Check sheet for the modelled part. Datum: model origin and axes. Units: mm. A direction names the side the tool comes from. Round coordinates to 2 decimals unless told otherwise and drop trailing zeros. Write each loop counter-clockwise with the first axis right and the second up, starting at its lowest first coordinate (ties: lowest second). Pieces come first, ordered by that corner, then holes. Notation, with made-up numbers: (-22.75, 29.5) -> (34.25, 29.5) arc R10 cw to (34.25, 33.5) -> close; hole circle Ø6 at (82, -40). An arc over 180 degrees is marked (long way). One line per item, written item: value.
from build123d import *

# Parameters (mm, degrees)
SKETCH1_W           = 30
SKETCH1_H           = 100
BOSS_EXTRUDE1_DEPTH = 3.75
CUT_EXTRUDE1_DEPTH  = 6.5


with BuildPart() as part:
    # Sketch1 → Boss-Extrude1 (new, symmetric)
    with BuildSketch(Plane(origin=(0, 0, 0), x_dir=(1, 0, 0), z_dir=(0, 1, 0))):
        with Locations((15, 0)):
            Rectangle(SKETCH1_W, SKETCH1_H)
    extrude(amount=BOSS_EXTRUDE1_DEPTH, both=True)

    # Sketch2 → Cut-Extrude1 (cut)
    with BuildSketch(Plane(origin=(0, -3.25, 0), x_dir=(1, 0, 0), z_dir=(0, 1, 0))):
        Polygon((0, 25), (0, -25), (15, -25.261825974), (15, 25.261825974), align=None)
    extrude(amount=CUT_EXTRUDE1_DEPTH, mode=Mode.SUBTRACT)


solid = part.part
Item 1: Mould release check, pull along Y, two halves, no side actions. Record for faces 1 (the flat face through (7, -3.25, 0)), 2 (the flat face through (15, 3.75, -1)), 3 (the flat face through (30, 0, 1)): pulls with the +Y half, pulls with the -Y half, needs draft (parallel to the pull), parting line crosses it, or undercut.
Answer:
face 1: undercut
face 2: pulls with the +Y half
face 3: needs draft
Item 2: Tool access check on faces 4 (the flat face through (15, 0, -50)), 5 (the flat face through (7, 3.25, 0)). Record the directions out of +Z, -Z, +X, -X, +Y, -Y that give a thin tool (end or side, any length) a straight path to the whole face; none if there is none.
Answer:
face 4: -Z, +X, -X, +Y, -Y
face 5: -X
Item 3: Sectioned sample at C-C on y = -0.25. Enter the section's corners in (x, z), and give its area (3 significant figures).
Answer:
outline: (0, -50) -> (30, -50) -> (30, 50) -> (0, 50) -> (0, 25) -> (15, 25.26) -> (15, -25.26) -> (0, -25) -> close
area: 2,250 mm^2
Item 4: Sectioned sample at B-B on z = -3. Enter the section's corners in (x, y), and give its area (4 significant figures).
Answer:
outline: (0, -3.75) -> (30, -3.75) -> (30, 3.75) -> (0, 3.75) -> (0, 3.25) -> (15, 3.25) -> (15, -3.25) -> (0, -3.25) -> close
area: 127.5 mm^2
Item 5: Sectioned sample at A-A on x = 6.5. Enter the section's corners in (y, z), and give its area (3 significant figures).
Answer:
outline: (-3.75, -50) -> (3.75, -50) -> (3.75, 50) -> (-3.75, 50) -> close; hole (-3.25, -25.11) -> (3.25, -25.11) -> (3.25, 25.11) -> (-3.25, 25.11) -> close
area: 424 mm^2
Item 6: Thickness scan on line 1 (X direction, y = 2, z = 15); line 2 (Z direction, x = 13.25, y = -1.5); line 3 (Z direction, x = 8.25, y = -0.25). Record the ranges inside material, lowest first.
Answer:
line 1: x = 15 to 30
line 2: z = -50 to -25.23, 25.23 to 50
line 3: z = -50 to -25.14, 25.14 to 50
